Part model, mm, in its own coordinate system. A direction names the side the tool comes from. Round coordinates to 2 decimals unless told otherwise and drop trailing zeros. Loops run counter-clockwise (first coordinate to the right, second up) from the corner with the lowest first, then second, coordinate; pieces in that order, holes last.
(1) Mould opens along Y. For faces 3 (the face through (2.54, 5.56, -7.6)), 4 (the face through (3, -65, 0)), 5 (the face through (5, -18, 0)) say: +Y half, -Y half, draft (parallel to the pull), parting line (faces both ways), or undercut.
(2) Tool access for faces 1 (the face through (2, 20, 0)), 2 (the face through (0, -18, 0)): list every direction of +Z, -Z, +X, -X, +Y, -Y with a clear straight run to the whole face (end or side of a thin tool).
(3) Probe probe 1 along Y at (x, z) = (3.9, 9); probe 2 along Y at (x, z) = (2.65, 0); probe 3 along Y at (x, z) = (1.35, -8). List the from-to ranges inside material, lowest first.
(4) Cut at B-B on x = 2.55. List the corners of the cut face in (y, z).
(5) Cut at A-A on z = 0. List the corners of the cut face in (x, y), then the cut area to 3 significant figures.
(6) Flat gauge pins, fed straight in: pin 1 (1.5 mm diameter, centred on x = 2.5, z = 18.5, fed in from +Y); pin 2 (2.5 mm diameter, centred on y = -5.5, z = -9, fed in from -X); pin 3 (2 mm diameter, centred on x = 3, y = 18, fed in from +Z); pin 4 (3 mm diameter, centred on x = 2, z = -1, fed in from +Y). Where does each tip first touch, or does it go through?
(7) Cut at D-D on z = 9. Count the separate pieces of the cut face and the enclosed holes in it, then the cut area to 3 significant figures.
(8) Cut at C-C on y = -5.5. List the corners of the cut face in (x, z).
from build123d import *

# Parameters (mm, degrees)
EXTRUDE_1_DEPTH     = 5
SKETCH_2_R          = 1.4
CUT_EXTRUDE_1_DEPTH = 5
CHAMFER_1_SIZE      = 1
SKETCH_4_W          = 22
SKETCH_4_H          = 7
CUT_EXTRUDE_4_DEPTH = 10
CHAMFER_2_SIZE      = 0.5


with BuildPart() as part:
    # 草图1 → 凸台-拉伸1 (new body)
    with BuildSketch(Plane(origin=(0, 0, 0), x_dir=(0, 0, -1), z_dir=(1, 0, 0))):
        with BuildLine():
            Line((-27.5, 0), (-27.5, -65))
            Line((-27.5, -65), (27.5, -65))
            Line((27.5, -65), (27.5, 0))
            ThreePointArc((27.5, 0), (0, 27.5), (-27.5, 0))
        make_face()
    extrude(amount=EXTRUDE_1_DEPTH)

    # 草图2 → 切除-拉伸1 (cut)
    with BuildSketch(Plane(origin=(5, 0, 0), x_dir=(0, 0, -1), z_dir=(1, 0, 0))):
        with Locations((-9, 5.5)):
            Circle(SKETCH_2_R)
        with Locations((9, 5.5)):
            Circle(SKETCH_2_R)
        with Locations((9, -5.5)):
            Circle(SKETCH_2_R)
        with Locations((-9, -5.5)):
            Circle(SKETCH_2_R)
    extrude(amount=-CUT_EXTRUDE_1_DEPTH, mode=Mode.SUBTRACT)

    # 倒角1
    chamfer_1_edges = [part.edges().sort_by_distance(p)[0] for p in [
        (0, -32.5, -27.5),
        (0, -65, 0),
        (0, -32.5, 27.5),
        (0, 27.5, 0),
    ]]
    chamfer(chamfer_1_edges, length=CHAMFER_1_SIZE)

    # 草图4 → 切除-拉伸4 (cut)
    with BuildSketch(Plane.ZY):
        with Locations((0, 16.5)):
            Rectangle(SKETCH_4_W, SKETCH_4_H)
    extrude(amount=-CUT_EXTRUDE_4_DEPTH, mode=Mode.SUBTRACT)

    # 倒角2
    chamfer_2_edges = [part.edges().sort_by_distance(p)[0] for p in [
        (5, 16.5, -11),
        (5, 20, 0),
        (5, 16.5, 11),
        (5, 13, 0),
        (0, 16.5, -11),
        (0, 13, 0),
        (0, 16.5, 11),
        (0, 20, 0),
    ]]
    chamfer(chamfer_2_edges, length=CHAMFER_2_SIZE)


solid = part.part
Final values:
1. face 3: undercut
1. face 4: -Y half
1. face 5: draft
2. face 1: +X, -X
2. face 2: +Z, -Z, -X, +Y, -Y
3. probe 1: y = -65 to -6.9, -4.1 to 4.1, 6.9 to 13, 20 to 25.99
3. probe 2: y = -65 to 13, 20 to 27.5
3. probe 3: y = -65 to -6.48, -4.52 to 4.52, 6.48 to 13, 20 to 26.31
4. outline: (-65, -27.5) - (0, -27.5) arc R27.5 ccw to (0, 27.5) - (-65, 27.5) - close; hole circle Ø2.8 at (-5.5, -9); hole circle Ø2.8 at (-5.5, 9); hole circle Ø2.8 at (5.5, -9); hole circle Ø2.8 at (5.5, 9); hole (13, -11) - (20, -11) - (20, 11) - (13, 11) - close
5. outline: (0, -64) - (1, -65) - (5, -65) - (5, 12.5) - (4.5, 13) - (0.5, 13) - (0, 12.5) - close; (0, 20.5) - (0.5, 20) - (4.5, 20) - (5, 20.5) - (5, 27.5) - (1, 27.5) - (0, 26.5) - close
5. area: 426 mm2
6. pin 1: stops at y = 21
6. pin 2: passes through
6. pin 3: stops at z = 21.62
6. pin 4: stops at y = 27.5
7. separate pieces: 4
7. enclosed holes: 0
7. area: 390 mm2
8. outline: (0, -26.5) - (1, -27.5) - (5, -27.5) - (5, -10.4) - (0, -10.4) - close; (0, -7.6) - (5, -7.6) - (5, 7.6) - (0, 7.6) - close; (0, 10.4) - (5, 10.4) - (5, 27.5) - (1, 27.5) - (0, 26.5) - close
